Source: CAD feature listing. Evaluate the final solid. Frame: model axes, mm. Give positions to 0.01 mm unless a question says otherwise; leave off trailing zeros. Write each loop counter-clockwise with the first axis right and the second up, starting at its lowest first coordinate (ties: lowest second). Pieces come first, ordered by that corner, then holes. Notation, with made-up numbers: (47.5, 77.5) -> (101.5, 77.5) arc R22 cw to (101.5, 102.5) -> close; hole circle Ø10 at (-40, 35). An arc over 180 degrees is marked (long way). Use one line per item in the form item = value. Start each with the question number.
(1) Material intervals for line 1 along Y through (x, z) = (0.25, 0.4); line 2 along Y through (x, z) = (8.25, 0.2); line 3 along Y through (x, z) = (5.75, 0.4), sorted ascending. Write a range as from..to.
(2) Draft query along X for faces 1 (the face through (6.963, 2.193, 0.493)), 2 (the face through (-10, -0.1, 0.5)), 3 (the face through (-0.1, -10, 0.5)). Return one class per face: pulls with the +X half, pulls with the -X half, needs draft (parallel to the pull), parting line crosses it, or undercut.
(3) Cut plane D-D, the plane y = 6.25. Output: boundary loops of the cut face in (x, z).
(4) Cut plane C-C, the plane x = -8.25. Output: boundary loops of the cut face in (y, z), and give its area (3 significant figures).
(5) Cut plane A-A, the plane x = 0. Output: boundary loops of the cut face in (y, z).
from build123d import *

# Parameters (mm, degrees)
SKETCH1_W           = 20
SKETCH1_H           = 20
SKETCH1_R           = 7.3
BOSS_EXTRUDE1_DEPTH = 1
SKETCH2_R           = 1.5
CUT_EXTRUDE1_DEPTH  = 1


with BuildPart() as part:
    # Sketch1 → Boss-Extrude1 (new body)
    with BuildSketch(Plane.XY):
        Rectangle(SKETCH1_W, SKETCH1_H)
        Circle(SKETCH1_R, mode=Mode.SUBTRACT)
    extrude(amount=BOSS_EXTRUDE1_DEPTH)

    # Sketch2 → Cut-Extrude1 (cut)
    with BuildSketch(Plane.XY.offset(1)):
        with Locations((-7.071067812, 7.071067812)):
            Circle(SKETCH2_R)
        with Locations((7.071067812, 7.071067812)):
            Circle(SKETCH2_R)
        with Locations((7.071067812, -7.071067812)):
            Circle(SKETCH2_R)
        with Locations((-7.071067812, -7.071067812)):
            Circle(SKETCH2_R)
    extrude(amount=-CUT_EXTRUDE1_DEPTH, mode=Mode.SUBTRACT)


solid = part.part
Geometry says:
q1.line_1 = -10..-7.3, 7.3..10
q1.line_2 = -10..-8, -6.14..6.14, 8..10
q1.line_3 = -10..-7.78, -6.36..-4.5, 4.5..6.36, 7.78..10
q2.face_1 = undercut
q2.face_2 = pulls with the -X half
q2.face_3 = needs draft
q3.outline = (-10, 0) -> (-8.33, 0) -> (-8.33, 1) -> (-10, 1) -> close; (-5.82, 0) -> (-3.77, 0) -> (-3.77, 1) -> (-5.82, 1) -> close; (3.77, 0) -> (5.82, 0) -> (5.82, 1) -> (3.77, 1) -> close; (8.33, 0) -> (10, 0) -> (10, 1) -> (8.33, 1) -> close
q4.outline = (-10, 0) -> (-8, 0) -> (-8, 1) -> (-10, 1) -> close; (-6.14, 0) -> (6.14, 0) -> (6.14, 1) -> (-6.14, 1) -> close; (8, 0) -> (10, 0) -> (10, 1) -> (8, 1) -> close
q4.area = 16.3 mm^2
q5.outline = (-10, 0) -> (-7.3, 0) -> (-7.3, 1) -> (-10, 1) -> close; (7.3, 0) -> (10, 0) -> (10, 1) -> (7.3, 1) -> close
